```python
from build123d import *

# Parameters (mm, degrees)
F1_DEPTH = 62.9
F2_DEPTH = 20
F3_START = -19.2
F3_DEPTH = 5.8
F4_W     = 17.40286313
F4_H     = 7.7177907806
F4_W_2   = 16.192227602
F4_H_2   = 9.8363999277
F4_W_3   = 17.4506753683
F4_H_3   = 12.9930109251


with BuildPart() as f1:
    # F0 (on Front) → F1 (new body)
    with BuildSketch(Plane.XZ):
        Polygon((-75.5699121067, 0), (0, 0), (0, 5.6038224138), (-94.5054218173, 5.6038224138), align=None)
        Polygon((-98.0191975832, 0), (-75.5699121067, 0), (-94.5054218173, 5.6038224138), (-98.0191975832, 5.6038224138), align=None)
    extrude(amount=F1_DEPTH)

    # F0 (on Front) → F2 (join)
    with BuildSketch(Plane.XZ):
        Polygon((0, -22.3643500358), (-75.5699121067, 0), (-98.0191975832, 0), (12.9512035679, -31.4862316811), (38.7845113873, -38.8160557302), (42.6020771265, -39.8992342902), (68.3070272207, -47.1926387081), (72.8881061077, -48.4924529801), (98.6080013494, -55.7900978655), (99.5356142521, -50.6061278284), align=None)
        Polygon((-98.0191975832, 0), (-75.5699121067, 0), (-94.5054218173, 5.6038224138), (-98.0191975832, 5.6038224138), align=None)
        Polygon((72.8881061077, -115.9313321114), (72.8881061077, -48.4924529801), (68.3070272207, -47.1926387081), (68.3070272207, -115.9313321114), align=None)
        Polygon((42.6020771265, -39.8992342902), (38.7845113873, -38.8160557302), (38.7845113873, -115.9313321114), (42.6020771265, -115.9313321114), align=None)
    extrude(amount=-F2_DEPTH)

    # F0 (on Front) → F3 (join)
    with BuildSketch(Plane.XZ.offset(F3_START)):
        Polygon((0, -22.3643500358), (0, 0), (-75.5699121067, 0), align=None)
        Polygon((-75.5699121067, 0), (0, 0), (0, 5.6038224138), (-94.5054218173, 5.6038224138), align=None)
        Polygon((-94.5054218173, 5.6038224138), (0, 5.6038224138), (0, 12.5394500792), (-98.0191975832, 12.5394500792), (-98.0191975832, 5.6038224138), align=None)
        Polygon((38.7845113873, -38.8160557302), (12.9512035679, -31.4862316811), (12.9512035679, -115.9313321114), (38.7845113873, -115.9313321114), align=None)
        Polygon((68.3070272207, -47.1926387081), (42.6020771265, -39.8992342902), (42.6020771265, -115.9313321114), (68.3070272207, -115.9313321114), align=None)
        Polygon((100.0360324979, -115.9313321114), (98.6080013494, -55.7900978655), (72.8881061077, -48.4924529801), (72.8881061077, -115.9313321114), align=None)
        Polygon((42.6020771265, -39.8992342902), (38.7845113873, -38.8160557302), (38.7845113873, -115.9313321114), (42.6020771265, -115.9313321114), align=None)
        Polygon((72.8881061077, -115.9313321114), (72.8881061077, -48.4924529801), (68.3070272207, -47.1926387081), (68.3070272207, -115.9313321114), align=None)
    extrude(amount=-F3_DEPTH)

    # F5: sweep along a path in F0
    with BuildLine(Plane.XZ) as f5_path:
        Line((99.5356142521, -50.6061278284), (98.6080013494, -55.7900978655))
    # F4 (on face) → F5 (sweep, cut)
    with BuildSketch(Plane(origin=(-5.872766279, 0, -20.6980383189), x_dir=(0.9620252097, 0, -0.2729606122), z_dir=(0.2729606122, 0, 0.9620252097))):
        with Locations((34.340926446, 6.8220865214)):
            Rectangle(F4_W, F4_H)
        with Locations((61.5801885724, 8.032720536)):
            Rectangle(F4_W_2, F4_H_2)
        with Locations((93.2230502367, 9.7836576169)):
            Rectangle(F4_W_3, F4_H_3)
    sweep(path=f5_path.line, mode=Mode.SUBTRACT)


solid = f1.part
```
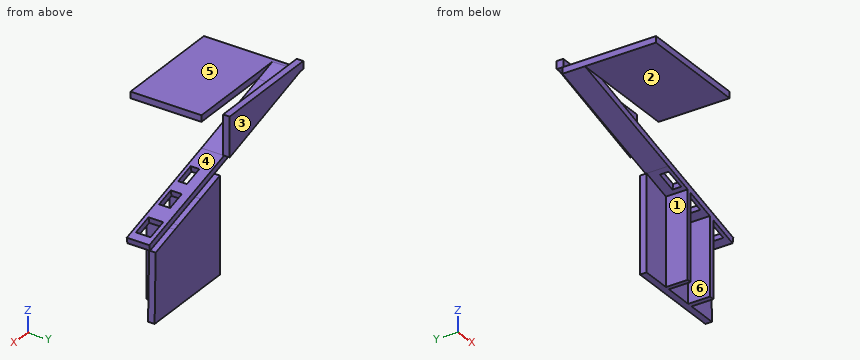
Input: part model. Units: mm. Frame: model coordinates. Face numbers are marked on the shaded views. A direction names the side the tool comes from. Give positions to 0.01 mm unless a question says otherwise; leave off trailing zeros. Loops run counter-clockwise (first coordinate to the right, second up) from the corner with the lowest first, then second, coordinate; pieces in that order, holes last. Notation, with made-up numbers: (-12.75, 17.25) -> (19.25, 17.25) arc R32 ccw to (19.25, 43.25) -> close; hole circle Ø11 at (-33, -36.75). An arc over 180 degrees is marked (long way). Use a Markdown table: item, result.
Q1. Section query B-B, the plane z = -10.5. Return the cut outline in (x, y).
Entries:
| item | result |
|---|---|
| outline | (-61.01, 0) -> (-40.09, 0) -> (-40.09, 19.2) -> (0, 19.2) -> (0, 25) -> (-40.09, 25) -> (-40.09, 20) -> (-61.01, 20) -> close |
Q2. Ray query, probe 1 along X at (y, z) = (8.5, -94.5); probe 2 along Y at (x, z) = (-49, -3.5); probe 3 along Z at (x, y) = (-9.5, -26). Return the intervals inside material, ascending. Write a range as from..to.
Entries:
| item | result |
|---|---|
| probe 1 | x = 38.78..42.6, 68.31..72.89 |
| probe 2 | y = 19.2..25 |
| probe 3 | z = 0..5.6 |
Q3. Section query C-C, the plane y = -13.5. Return the cut outline in (x, z), plus the area to 3 significant figures.
Entries:
| item | result |
|---|---|
| outline | (-98.02, 0) -> (0, 0) -> (0, 5.6) -> (-98.02, 5.6) -> close |
| area | 549 mm² |
Q4. Section query D-D, the plane x = -38. Return the cut outline in (y, z).
Entries:
| item | result |
|---|---|
| outline | (-62.9, 0) -> (0, 0) -> (0, 5.6) -> (-62.9, 5.6) -> close; (0, -17.03) -> (20, -17.03) -> (20, -11.12) -> (25, -11.12) -> (25, 12.54) -> (19.2, 12.54) -> (19.2, -11.12) -> (0, -11.12) -> close |
Q5. Pull-direction query (X, two-part tool) for the marked faces 4, 5 and 6; classes: pulls with the +X half, pulls with the -X half, needs draft (parallel to the pull), parting line crosses it, or undercut.
Entries:
| item | result |
|---|---|
| face 4 | pulls with the +X half |
| face 5 | needs draft |
| face 6 | undercut |
Q6. Section query A-A, the plane x = 84. Return the cut outline in (y, z).
Entries:
| item | result |
|---|---|
| outline | (0, -51.65) -> (3.29, -51.65) -> (3.29, -46.2) -> (0, -46.2) -> close; (16.28, -51.65) -> (19.2, -51.65) -> (19.2, -115.93) -> (25, -115.93) -> (25, -51.65) -> (20, -51.65) -> (20, -46.2) -> (16.28, -46.2) -> close |
Q7. First-contact query: P1, Ø15.5, axis at y = 9, z = -75, coming from the -X side; P2, Ø3, axis at x = 25.5, z = -35, coming from the -Y side; P3, Ø3, axis at x = 30, z = -34, coming from the +Y side. Flat tips, straight axial feed; report the tip coordinate or a pass-through.
Entries:
| item | result |
|---|---|
| P1 | stops at x = 38.78 |
| P2 | stops at y = 0 |
| P3 | stops at y = 20 |
Q8. Access query for the marked faces 1, 2 and 3. Directions: +Z, -Z, +X, -X, +Y, -Y. A direction counts if a zero-diameter tool reaches every point of the face in a straight line with its end or side. Return the directions, or none.
Entries:
| item | result |
|---|---|
| face 1 | -Z, -X, -Y |
| face 2 | -Z, +X, -X, -Y |
| face 3 | +Z, -Z, +X, -X, +Y |
